Autodesk Inventor part; units mm, degrees
ref_plane "YZ Plane" through (0, 0, 0) normal (1, 0, 0) x (0, 1, 0)
ref_plane "XZ Plane" through (0, 0, 0) normal (0, 1, 0) x (-1, 0, 0)
ref_plane "XY Plane" through (0, 0, 0) normal (0, 0, 1) x (1, 0, 0)
sketch "草圖1" plane through (0, 0, 0) normal (0, 1, 0) x (-1, 0, 0)
  line L0 (5, 7.5) -> (-5, 7.5)
  line L1 (-5, 7.5) -> (-5, -7.5)
  line L2 (-5, -7.5) -> (5, -7.5)
  line L3 (5, -7.5) -> (5, 7.5)
  point P0 (0, 0)
  point P1 (5, 0)
  point P2 (0, -7.5)
  dimension "d0" = 10
  dimension "d1" = 15
extrude "擠出1" add sketch "草圖1" along normal blind 2
sketch "草圖2" plane through (0, 0, 0) normal (0, -1, 0) x (1, 0, 0)
  line L0 (5, 7.5) -> (5, -7.5)
  line L1 (-5, 7.5) -> (5, 7.5)
  line L2 (-5, -7.5) -> (-5, 7.5)
  line L3 (5, -7.5) -> (-5, -7.5)
  circle A0 centre (2.5, 5) radius 1.25
  circle A1 centre (2.5, 5) radius 2.5
  point P0 (0, 0)
  dimension "d4" = 2.5
  dimension "d5" = 5
  dimension "d6" = 2.5
  dimension "d7" = 2.5
extrude "擠出2" cut sketch "草圖2" against normal blind 1.5 contours A0
pattern_linear "矩形陣列1" count 3 spacing 5 along (0, 0, -1) count 2 spacing 5 along (-1, 0, 0) of "擠出2"
sketch "草圖3" plane through (0, 2, 0) normal (0, 1, 0) x (1, 0, 0)
  circle A0 centre (2.5, -5) radius 1.7
  line L0 (5, -7.5) -> (5, 7.5)
  line L1 (-5, -7.5) -> (5, -7.5)
  point P0 (0, 0)
  dimension "d16" = 3.4
  dimension "d17" = 2.5
  dimension "d18" = 2.5
extrude "擠出3" add sketch "草圖3" along normal blind 1.5
pattern_linear "矩形陣列2" count 3 spacing 5 along (0, 0, -1) count 2 spacing 5 along (-1, 0, 0) of "擠出3"
properties part number "110033226_ipt_02_草地一"
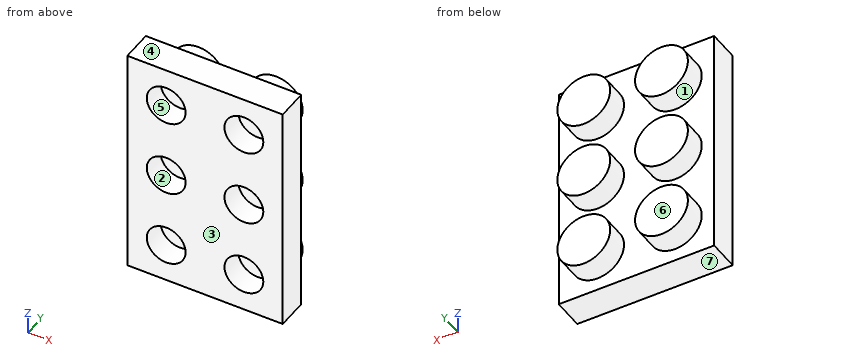
Read the model definition and answer for the solid it produces. Units are mm, in the model's axes. Face numbers are marked on the shaded views. A direction names the side the tool comes from. Round coordinates to 2 decimals unless told otherwise and drop trailing zeros. Write each loop counter-clockwise with the first axis right and the second up, starting at its lowest first coordinate (ties: lowest second). Pieces come first, ordered by that corner, then holes. Notation, with made-up numbers: (-13, 44) -> (46, 44) arc R16 cw to (46, 60) -> close; hole circle Ø4 at (-18, 31). An arc over 180 degrees is marked (long way). Answer in a Markdown table with one row per item. Add a question column.
1) Find section B-B, the plane y = 2.8. Determine the outline of the cut face in (x, z), and give its area (3 significant figures).
2) Find section A-A, the plane y = 0.8. Determine the outline of the cut face in (x, z), and give its area (3 significant figures).
3) Find section D-D, the plane z = 0.5. Determine the outline of the cut face in (x, y).
4) Consider line 1 (Z direction, x = 2.5, y = 0.4); line 2 (Z direction, x = 3.5, y = 3.1); line 3 (Z direction, x = 1.5, y = 0.6). Determine where each line is inside the solid, lowest interval first.
5) Which of the six approach directions +Z, -Z, +X, -X, +Y, -Y give full straight-line access (tool end or side, diameter ignored) to the marked faces 1, 2 and 3?
6) Determine the mould class of the marked faces 4, 5, 6 and 7 for opening direction Z: pulls with the +Z half, pulls with the -Z half, needs draft (parallel to the pull), parting line crosses it, or undercut.
7) Given P1, Ø0.8, axis at x = -2.5, z = -4.5, coming from the -Y side; P2, Ø1, axis at x = 1, z = 3, coming from the +Y side, each flat-ended and moving along its own axis, determine where each tip first touches the part or whether it passes through.
8) Find section C-C, the plane x = -4. Determine the outline of the cut face in (y, z).
Findings below:
| question | item | result |
|---|---|---|
| 1 | outline | circle Ø3.4 at (-2.5, -5); circle Ø3.4 at (-2.5, 0); circle Ø3.4 at (-2.5, 5); circle Ø3.4 at (2.5, -5); circle Ø3.4 at (2.5, 0); circle Ø3.4 at (2.5, 5) |
| 1 | area | 54.5 mm² |
| 2 | outline | (-5, -7.5) -> (5, -7.5) -> (5, 7.5) -> (-5, 7.5) -> close; hole circle Ø2.5 at (-2.5, -5); hole circle Ø2.5 at (-2.5, 0); hole circle Ø2.5 at (-2.5, 5); hole circle Ø2.5 at (2.5, -5); hole circle Ø2.5 at (2.5, 0); hole circle Ø2.5 at (2.5, 5) |
| 2 | area | 121 mm² |
| 3 | outline | (-5, 0) -> (-3.65, 0) -> (-3.65, 1.5) -> (-1.35, 1.5) -> (-1.35, 0) -> (1.35, 0) -> (1.35, 1.5) -> (3.65, 1.5) -> (3.65, 0) -> (5, 0) -> (5, 2) -> (4.12, 2) -> (4.12, 3.5) -> (0.88, 3.5) -> (0.88, 2) -> (-0.88, 2) -> (-0.88, 3.5) -> (-4.12, 3.5) -> (-4.12, 2) -> (-5, 2) -> close |
| 4 | line 1 | -7.5 to -6.25, -3.75 to -1.25, 1.25 to 3.75, 6.25 to 7.5 |
| 4 | line 2 | -6.37 to -3.63, -1.37 to 1.37, 3.63 to 6.37 |
| 4 | line 3 | -7.5 to -5.75, -4.25 to -0.75, 0.75 to 4.25, 5.75 to 7.5 |
| 5 | face 1 | +Y |
| 5 | face 2 | -Y |
| 5 | face 3 | +Z, -Z, +X, -X, -Y |
| 6 | face 4 | pulls with the +Z half |
| 6 | face 5 | undercut |
| 6 | face 6 | needs draft |
| 6 | face 7 | pulls with the -Z half |
| 7 | P1 | y = 1.5 |
| 7 | P2 | y = 2 |
| 8 | outline | (0, -7.5) -> (2, -7.5) -> (2, -5.8) -> (3.5, -5.8) -> (3.5, -4.2) -> (2, -4.2) -> (2, -0.8) -> (3.5, -0.8) -> (3.5, 0.8) -> (2, 0.8) -> (2, 4.2) -> (3.5, 4.2) -> (3.5, 5.8) -> (2, 5.8) -> (2, 7.5) -> (0, 7.5) -> close |
